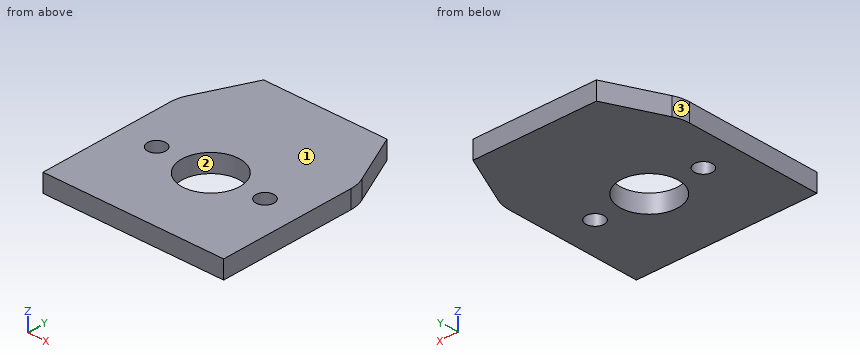
```python
from build123d import *

# Parameters (mm, degrees)
SKETCH1_R           = 8
SKETCH1_R_2         = 2.5
BOSS_EXTRUDE1_DEPTH = 2.5


with BuildPart() as part:
    # Sketch1 → Boss-Extrude1 (new, symmetric)
    with BuildSketch(Plane.XY):
        with BuildLine():
            Line((-25, 0), (-25, 37.783053374))
            ThreePointArc((-25, 37.783053374), (-24.762960071, 39.947449513), (-24.06307787, 42.009235991))
            Line((-24.06307787, 42.009235991), (-17.072769811, 57))
            Line((-17.072769811, 57), (17.072769811, 57))
            Line((17.072769811, 57), (24.06307787, 42.009235991))
            ThreePointArc((24.06307787, 42.009235991), (24.762960071, 39.947449513), (25, 37.783053374))
            Line((25, 37.783053374), (25, 0))
            Line((25, 0), (-25, 0))
        make_face()
        with Locations((0, 23)):
            Circle(SKETCH1_R, mode=Mode.SUBTRACT)
        with Locations((-15, 23)):
            Circle(SKETCH1_R_2, mode=Mode.SUBTRACT)
        with Locations((15, 23)):
            Circle(SKETCH1_R_2, mode=Mode.SUBTRACT)
    extrude(amount=BOSS_EXTRUDE1_DEPTH, both=True)


solid = part.part
```
Design review of the part built by this model. Coordinates are the model's own, in mm. Face numbers are marked on the shaded views. Round coordinates to 2 decimals unless told otherwise and drop trailing zeros. Write each loop counter-clockwise with the first axis right and the second up, starting at its lowest first coordinate (ties: lowest second). Pieces come first, ordered by that corner, then holes. Notation, with made-up numbers: (39, -34.5) -> (53, -34.5) arc R21 ccw to (53, -1.5) -> close; hole circle Ø11 at (50, 15). An arc over 180 degrees is marked (long way). Answer in a Markdown table with one row per item.
Q1. Take a section at D-D, the plane x = 0. State the section outline as (y, z) points, then the cut area to 3 significant figures.
The answers:
| item | result |
|---|---|
| outline | (0, -2.5) -> (15, -2.5) -> (15, 2.5) -> (0, 2.5) -> close; (31, -2.5) -> (57, -2.5) -> (57, 2.5) -> (31, 2.5) -> close |
| area | 205 mm² |
Q2. Draft analysis for pull direction Y (two halves, no side actions). For the marked faces 1, 2 and 3, state which applies: +Y half, -Y half, draft (parallel to the pull), parting line (faces both ways), or undercut.
The answers:
| item | result |
|---|---|
| face 1 | draft |
| face 2 | undercut |
| face 3 | +Y half |
Q3. To check wall thickness, follow L1, parallel to Y at x = 15, z = -0.8; L2, parallel to Y at x = 0, z = 0.25; L3, parallel to X at y = 27, z = -1.9. State the ranges of each line that lie inside material, in increasing order. Write a range as [from, to].
The answers:
| item | result |
|---|---|
| L1 | [0, 20.5], [25.5, 57] |
| L2 | [0, 15], [31, 57] |
| L3 | [-25, -6.93], [6.93, 25] |
Q4. Clearance check with a flat-ended pin moving along its axis: pin 1 Ø1.5 at (x, y) = (13.5, 23.5) entering from +Z. State where the tip first meets the part, or that it passes through.
The answers:
| item | result |
|---|---|
| pin 1 | through |
Q5. Take a section at B-B, the plane x = 15. State the section outline as (y, z) points.
The answers:
| item | result |
|---|---|
| outline | (0, -2.5) -> (20.5, -2.5) -> (20.5, 2.5) -> (0, 2.5) -> close; (25.5, -2.5) -> (57, -2.5) -> (57, 2.5) -> (25.5, 2.5) -> close |
Q6. Take a section at A-A, the plane z = 0.4. State the section outline as (x, y) points, then the cut area to 3 significant figures.
The answers:
| item | result |
|---|---|
| outline | (-25, 0) -> (25, 0) -> (25, 37.78) arc R10 ccw to (24.06, 42.01) -> (17.07, 57) -> (-17.07, 57) -> (-24.06, 42.01) arc R10 ccw to (-25, 37.78) -> close; hole circle Ø5 at (-15, 23); hole circle Ø16 at (0, 23); hole circle Ø5 at (15, 23) |
| area | 2,470 mm² |
Q7. Take a section at C-C, the plane y = 23. State the section outline as (x, z) points, then the cut area to 3 significant figures.
The answers:
| item | result |
|---|---|
| outline | (-25, -2.5) -> (-17.5, -2.5) -> (-17.5, 2.5) -> (-25, 2.5) -> close; (-12.5, -2.5) -> (-8, -2.5) -> (-8, 2.5) -> (-12.5, 2.5) -> close; (8, -2.5) -> (12.5, -2.5) -> (12.5, 2.5) -> (8, 2.5) -> close; (17.5, -2.5) -> (25, -2.5) -> (25, 2.5) -> (17.5, 2.5) -> close |
| area | 120 mm² |
